from build123d import *

# Parameters (mm, degrees)
F0_W      = 60
F0_H      = 40
F1_DEPTH  = 10
F2_W      = 60
F2_H      = 10
F3_DEPTH  = 30
F4_W      = 20
F4_H      = 10
F5_DEPTH  = 20
F6_R      = 19.99999
F8_DEPTH  = 10
F9_W      = 20
F9_H      = 10
F10_DEPTH = 20
F12_DEPTH = 10


# Not quite as in the source:
# - a fillet or chamfer is up to 0.001 mm smaller than in the source, because OpenCascade refuses the exact size


with BuildPart() as f1:
    # F0 (on Top) → F1 (new body)
    with BuildSketch(Plane.XY):
        with Locations((-2.2019557655, 9.2856339355)):
            Rectangle(F0_W, F0_H)
    extrude(amount=F1_DEPTH)

    # F2 (on face) → F3 (join)
    with BuildSketch(Plane.XY.offset(10)):
        with Locations((-2.2019557655, 24.2856339355)):
            Rectangle(F2_W, F2_H)
    extrude(amount=F3_DEPTH)

    # F4 (on face) → F5 (cut)
    with BuildSketch(Plane.XY.offset(40)):
        with Locations((-22.2019557655, 24.2856339355)):
            Rectangle(F4_W, F4_H)
    extrude(amount=-F5_DEPTH, mode=Mode.SUBTRACT)

    # F6 (radius 20 in the source; OpenCascade refuses exactly that, so slightly less here)
    f6_edges = [f1.edges().sort_by_distance(p)[0] for p in [
        (-12.201956, 24.285634, 40),
        (27.798044, 24.285634, 40),
    ]]
    fillet(f6_edges, radius=F6_R)

    # F7 (on face) → F8 (cut)
    with BuildSketch(Plane.XZ.offset(-19.2856339355)):
        with BuildLine():
            ThreePointArc((7.7980442039, 10), (14.8691120356, 12.9289321773), (17.7980442345, 20))
            ThreePointArc((17.7980442345, 20), (0.7269764335, 27.0710678227), (7.7980442039, 10))
        make_face()
    extrude(amount=-F8_DEPTH, mode=Mode.SUBTRACT)

    # F9 (on face) → F10 (join)
    with BuildSketch(Plane.XY.offset(10)):
        with Locations((-22.2019557655, -5.7143660645)):
            Rectangle(F9_W, F9_H)
    extrude(amount=F10_DEPTH)

    # F11 (on face) → F12 (cut)
    with BuildSketch(Plane.XZ.offset(10.7143660645)):
        with BuildLine():
            Line((-12.2019557655, 30), (-22.2019557655, 30))
            ThreePointArc((-22.2019557655, 30), (-19.2730235774, 22.9289321881), (-12.2019557655, 20))
            Line((-12.2019557655, 20), (-12.2019557655, 30))
        make_face()
    extrude(amount=-F12_DEPTH, mode=Mode.SUBTRACT)


solid = f1.part
Geometry check sheet. Reference: the model listing, model coordinates, mm. A direction names the side the tool comes from. Give positions to 0.01 mm unless a question says otherwise; leave off trailing zeros. Loops run counter-clockwise (first coordinate to the right, second up) from the corner with the lowest first, then second, coordinate; pieces in that order, holes last. Notation, with made-up numbers: M 22,87 L 33,87 A12 cw 33,96 Z; hole C 13.5,-21 d6. An arc over 180 degrees is marked long. Answer as a JSON object with one key per item and string values. Group by question number.
Item 1: Mould release check, pull along Y, two halves, no side actions. Record for faces 1 (the flat face through (-3, 29.286, 15)), 2 (the flat face through (27.798, 13, 8)), 3 (the flat face through (-25, -0.714, 18)), 4 (the flat face through (-3, 19.286, 21)): pulls with the +Y half, pulls with the -Y half, needs draft (parallel to the pull), parting line crosses it, or undercut.
Item 2: Material ranges on L1, parallel to Y at x = -23.5, z = 19.5; L2, parallel to Y at x = 5.5, z = 31; L3, parallel to Y at x = -23, z = 21.5, recorded low to high.
Item 3: Gauge pin test, flat ends, axial feed: pin 1 (3 mm diameter, centred on x = 19.5, z = 16, fed in from -Y); pin 2 (12 mm diameter, centred on y = 20, z = 35.5, fed in from +X); pin 3 (2 mm diameter, centred on x = -19.5, y = 14, fed in from +Z). Record the tip position at first contact, or that the pin passes through.
Item 4: Sectioned sample at A-A on x = 12. Record the boundary of the cut face in (y, z), plus the area to 3 significant figures.
Item 5: Sectioned sample at D-D on x = 5. Record the boundary of the cut face in (y, z), plus the area to 3 significant figures.
Item 6: Access from +Z, -Z, +X, -X, +Y, -Y to the whole of each face (thin tool, end or side, straight path). Record for faces 5 (the flat face through (-22, 24, 20)), 6 (the flat face through (-12.202, -6, 15)), 7 (the flat face through (-3, 10, 0)).
Item 7: Sectioned sample at B-B on z = 13.5. Record the boundary of the cut face in (x, y), plus the area to 3 significant figures.
Findings below:
{
 "1": {"face 1": "pulls with the +Y half", "face 2": "needs draft", "face 3": "undercut", "face 4": "pulls with the -Y half"},
 "2": {"L1": "-10.71 to -0.71, 19.29 to 29.29", "L2": "19.29 to 29.29", "L3": "-10.71 to -0.71"},
 "3": {"pin 1": "y = 19.29", "pin 2": "x = 25.4", "pin 3": "z = 10"},
 "4": {"outline": "M -10.71,0 L 29.29,0 L 29.29,10.93 L 19.29,10.93 L 19.29,10 L -10.71,10 Z; M 19.29,29.07 L 29.29,29.07 L 29.29,39.55 L 19.29,39.55 Z", "area": "514 mm2"},
 "5": {"outline": "M -10.71,0 L 29.29,0 L 29.29,10.4 L 19.29,10.4 L 19.29,10 L -10.71,10 Z; M 19.29,29.6 L 29.29,29.6 L 29.29,39.8 L 19.29,39.8 Z", "area": "506 mm2"},
 "6": {"face 5": "+Z, -X, +Y", "face 6": "+Z, +X, -Y", "face 7": "-Z, +X, -X, +Y, -Y"},
 "7": {"outline": "M -32.2,-10.71 L -12.2,-10.71 L -12.2,-0.71 L -32.2,-0.71 Z; M -32.2,19.29 L 0.2,19.29 L 0.2,29.29 L -32.2,29.29 Z; M 15.4,19.29 L 27.8,19.29 L 27.8,29.29 L 15.4,29.29 Z", "area": "648 mm2"}
}
